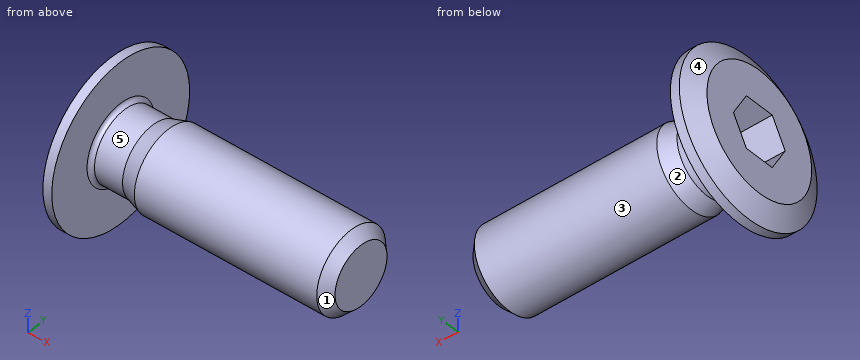
```python
from build123d import *

# Parameters (mm, degrees)
CUT_EXTRUDE1_DEPTH = 1.2


with BuildPart() as part:
    # Sketch1 → Revolve1 (revolve)
    with BuildSketch(Plane.XY):
        with BuildLine():
            Line((-0.5, 0), (-0.5, 1.52))
            Line((-0.5, 1.52), (-0.222871871, 2))
            Line((-0.222871871, 2), (0, 2))
            Line((0, 2), (0, 0.97725))
            ThreePointArc((0, 0.97725), (0.029289322, 0.906539322), (0.1, 0.87725))
            Line((0.1, 0.87725), (0.8, 0.87725))
            Line((0.8, 0.87725), (1.2, 1))
            Line((1.2, 1), (5.7545, 1))
            Line((5.7545, 1), (6, 0.7545))
            Line((6, 0.7545), (6, 0))
            Line((6, 0), (-0.5, 0))
        make_face()
    revolve(axis=Axis((6, 0, 0), (-1, 0, 0)))

    # Sketch2 → Cut-Revolve1 (revolve, cut)
    with BuildSketch(Plane.XY):
        Polygon((-0.5, 0), (-0.5, 0.65), (0.7, 0.65), (1.075277675, 0), align=None)
    revolve(axis=Axis((1.075277675, 0, 0), (-1, 0, 0)), mode=Mode.SUBTRACT)

    # Sketch3 → Cut-Extrude1 (cut)
    with BuildSketch(Plane(origin=(-0.5, 0, 0), x_dir=(0, 0, -1), z_dir=(1, 0, 0))):
        Polygon((-0.65, -0.375277675), (0, -0.75055535), (0.65, -0.375277675), (0.65, 0.375277675), (0, 0.75055535), (-0.65, 0.375277675), align=None)
    extrude(amount=CUT_EXTRUDE1_DEPTH, mode=Mode.SUBTRACT)


solid = part.part
```
CAD build for the part. Positions are in the model's coordinates, mm. Face numbers are marked on the shaded views. A direction names the side the tool comes from. Give positions to 0.01 mm unless a question says otherwise; leave off trailing zeros. Order: outer loops, then holes, each group sorted by start corner. A loop starts at its lowest first (then second) coordinate and runs counter-clockwise, first axis right, second up.
(1) Tool access for the marked faces 1 and 2: list every direction of +Z, -Z, +X, -X, +Y, -Y with a clear straight run to the whole face (end or side of a thin tool).
(2) Drill centre lines: L1, parallel to X at y = 1.1, z = -0.45; L2, parallel to Z at x = 4.5, y = -0.2; L3, parallel to Z at x = 0.5, y = 0.45. Where is each one in solid material? Low to high.
(3) Saw through at A-A, the plane x = 3.25. Give the cut face in (y, z), then the cut area to 3 significant figures.
(4) Mould opens along X. For the marked faces 3, 4 and 5 say: released by +X, released by -X, zero draft, split by the parting line, or undercut.
(5) Flat gauge pin, fed straight in: pin 1 (1.5 mm diameter, centred on x = 5, z = -1.5, fed in from +Y). Where does the tip first touch, or does it go through?
Results found:
1. face 1: +X
1. face 2: none
2. L1: x = -0.5 to 0
2. L2: z = -0.98 to 0.98
2. L3: z = -0.75 to -0.52, 0.52 to 0.75
3. outline: circle Ø2 at (0, 0)
3. area: 3.14 mm2
4. face 3: zero draft
4. face 4: released by -X
4. face 5: undercut
5. pin 1: stops at y = 0.66
